The model under review builds one solid part; all positions refer to its coordinate system, in mm. A direction names the side the tool comes from. Give positions to 0.01 mm unless a question says otherwise; leave off trailing zeros. Order: outer loops, then holes, each group sorted by start corner. A loop starts at its lowest first (then second) coordinate and runs counter-clockwise, first axis right, second up. Notation, with made-up numbers: (52.25, 45) - (58.25, 45) arc R21 cw to (58.25, 64) - close; hole circle Ø11 at (-35.75, 71). An arc over 180 degrees is marked (long way). Use CSV: the item, a comma, the result in double quotes.
Autodesk Inventor part; units mm, degrees
ref_plane "YZ Plane" through (0, 0, 0) normal (1, 0, 0) x (0, 1, 0)
ref_plane "XZ Plane" through (0, 0, 0) normal (0, 1, 0) x (-1, 0, 0)
ref_plane "XY Plane" through (0, 0, 0) normal (0, 0, 1) x (1, 0, 0)
sketch "Sketch1" plane through (0, 0, 0) normal (0, 0, 1) x (1, 0, 0)
  line L0 (0, 0) -> (25.4, 0)
  line L1 (25.4, 76.2) -> (0, 76.2)
  line L2 (0, 76.2) -> (0, 0)
  line L3 (25.4, 3.175) -> (3.175, 3.175)
  line L4 (3.175, 3.175) -> (3.175, 73.025)
  line L5 (3.175, 73.025) -> (25.4, 73.025)
  line L6 (25.4, 0) -> (25.4, 3.175)
  line L7 (25.4, 73.025) -> (25.4, 76.2)
  dimension "d0" = 76.2
  dimension "d1" = 25.4
  dimension "d2" = 3.175
  dimension "d3" = 3.175
  dimension "d4" = 3.175
extrude "Extrusion1" add sketch "Sketch1" along normal blind 939.8
sketch "Sketch2" plane through (0, 76.2, 0) normal (0, 1, 0) x (1, 0, 0)
  line L0 (0, -939.8) -> (25.4, -939.8)
  line L1 (25.4, 0) -> (25.4, -939.8)
  line L2 (25.4, 0) -> (0, 0)
  line L3 (0, 0) -> (0, -939.8)
  line L4 (0, -939.8) -> (25.4, -914.4)
  line L5 (0, 0) -> (25.4, -25.4)
  line L6 (3.175, -936.625) -> (3.175, -771.525)
  line L7 (3.175, -771.525) -> (25.4, -771.525)
  line L8 (3.175, -3.175) -> (3.175, -168.275)
  line L9 (3.175, -168.275) -> (25.4, -168.275)
  dimension "d7" = 45
  dimension "d8" = 3.175
  dimension "d9" = 165.1
  dimension "d10" = 165.1
extrude "Extrusion2" cut sketch "Sketch2" against normal through all contours L4 L1 L0 | L2 L1 L5
extrude "Extrusion3" cut sketch "Sketch2" against normal up to next contours L6 L7 L1 L4 | L5 L1 L9 L8
sketch "Sketch3" plane through (0, 76.2, 939.8) normal (0, 1, 0) x (1, 0, 0)
  line L0 (25.4, 771.525) -> (25.4, 168.275)
  line L1 (25.4, 454.025) -> (3.175, 454.025)
  line L2 (3.175, 454.025) -> (3.175, 485.775)
  line L3 (3.175, 485.775) -> (25.4, 485.775)
  line L4 (25.4, 485.775) -> (25.4, 454.025)
  point P0 (0, 0)
  dimension "d15" = 31.75
  dimension "d16" = 22.225
  dimension "d17" = 454.025
extrude "Extrusion4" cut sketch "Sketch3" against normal blind 25.4
equation "\"d3\" = d2"
equation "\"d4\" = d2"
equation "\"d10\" = d9"
properties part number "frame U 1 by 3 long 2"
Item 1: Take a section at A-A, the plane x = 7.5. Give the boundary of the cut face in (y, z) (3 decimals), and give its area (3 significant figures).
Results list:
outline,"(0, 7.5) - (3.175, 7.5) - (3.175, 932.3) - (0, 932.3) - close; (73.025, 168.275) - (76.2, 168.275) - (76.2, 454.025) - (73.025, 454.025) - close; (73.025, 485.775) - (76.2, 485.775) - (76.2, 771.525) - (73.025, 771.525) - close"
area,"4,750 mm2"
Item 2: Mouldability with a two-part tool opening along Y and no side actions: class faces 1 (the face through (2.3, 29.8, 937.5)), 2 (the face through (13, 0, 463)), 3 (the face through (14, 73.025, 627)) as pulls with the +Y half, pulls with the -Y half, needs draft (parallel to the pull), parting line crosses it, or undercut.
Results list:
face 1,"needs draft"
face 2,"pulls with the -Y half"
face 3,"undercut"
Item 3: Tool access review of faces 4 (the face through (2, 30, 2)), 5 (the face through (14, 3.175, 463)): name each direction out of +Z, -Z, +X, -X, +Y, -Y from which nothing blocks a thin tool from reaching the whole face with its end or side.
Results list:
face 4,"-Z, +X, +Y, -Y"
face 5,"+Z, -Z, +X"
Item 4: Clearance check with flat-ended pins moving along their axes: pin 1 (1.6 mm diameter, centred on x = 19, y = 74.5, fed in from -Z) (3 decimals); pin 2 (3.5 mm diameter, centred on x = 12.5, y = 75, fed in from +Z) (3 decimals). State where each tip first meets the part, or that it passes through.
Results list:
pin 1,"stops at z = 168.275"
pin 2,"stops at z = 771.525"
Item 5: Wall thickness on L1, parallel to Y at x = 3.75, z = 453.5 (3 decimals); L2, parallel to X at y = 71.5, z = 70 (3 decimals): over which ranges is each line inside the solid? List them lowest first.
Results list:
L1,"y = 0 to 3.175, 73.025 to 76.2"
L2,"x = 0 to 3.175"
Item 6: Take a section at C-C, the plane y = 18.5. Give the boundary of the cut face in (x, z) (3 decimals).
Results list:
outline,"(0, 0) - (3.175, 3.175) - (3.175, 936.625) - (0, 939.8) - close"
Item 7: Take a section at D-D, the plane z = 77.5. Give the boundary of the cut face in (x, y) (3 decimals), and give its area (4 significant figures).
Results list:
outline,"(0, 0) - (25.4, 0) - (25.4, 3.175) - (3.175, 3.175) - (3.175, 76.2) - (0, 76.2) - close"
area,"312.5 mm2"
Item 8: Take a section at B-B, the plane z = 646. Give the boundary of the cut face in (x, y) (3 decimals), and give its area (3 significant figures).
Results list:
outline,"(0, 0) - (25.4, 0) - (25.4, 3.175) - (3.175, 3.175) - (3.175, 73.025) - (25.4, 73.025) - (25.4, 76.2) - (0, 76.2) - close"
area,"383 mm2"
